Autodesk Inventor part; units mm, degrees
ref_plane "YZ Plane" through (0, 0, 0) normal (1, 0, 0) x (0, 1, 0)
ref_plane "XZ Plane" through (0, 0, 0) normal (0, 1, 0) x (-1, 0, 0)
ref_plane "XY Plane" through (0, 0, 0) normal (0, 0, 1) x (1, 0, 0)
sketch "TFT LCD Touch Screen" plane through (0, 0, 0) normal (0, 0, 1) x (1, 0, 0)
  line L0 (-55, 32.5) -> (55, 32.5)
  line L1 (55, 32.5) -> (55, -32.5)
  line L2 (55, -32.5) -> (-55, -32.5)
  line L3 (-55, -32.5) -> (-55, 32.5)
  circle A0 centre (-51, 28.5) radius 1.5
  circle A1 centre (-51, -28.5) radius 1.5
  circle A2 centre (51, -28.5) radius 1.5
  circle A3 centre (51, 28.5) radius 1.5
  line L4 (-40, 29) -> (40, 29)
  line L5 (40, 29) -> (40, -29)
  line L6 (40, -29) -> (-40, -29)
  line L7 (-40, -29) -> (-40, 29)
  point P0 (0.75, 3.075)
  point P1 (0, 32.5)
  point P2 (55, 0)
  point P3 (0, 29)
  point P4 (-40, 0)
  dimension "d9" = 110
  dimension "d10" = 65
  dimension "d11" = 3
  dimension "d12" = 57
  dimension "d13" = 102
  dimension "d14" = 4
  dimension "d15" = 4
  dimension "d16" = 80
  dimension "d17" = 58
sketch "Hinges Screw Holes" plane through (0, 0, 0) normal (0, 0, 1) x (1, 0, 0)
  arc A0 (172, 94.429) -> (172, 97.929) centre (172, 96.179) ccw
  arc A1 (172, 68.929) -> (172, 72.429) centre (172, 70.679) ccw
  arc A2 (172, -27.2) -> (172, -23.7) centre (172, -25.45) ccw
  arc A3 (172, -52.7) -> (172, -49.2) centre (172, -50.95) ccw
  arc A4 (167, 97.929) -> (167, 94.429) centre (167, 96.179) ccw
  arc A5 (167, 72.429) -> (167, 68.929) centre (167, 70.679) ccw
  arc A6 (167, -23.7) -> (167, -27.2) centre (167, -25.45) ccw
  arc A7 (167, -49.2) -> (167, -52.7) centre (167, -50.95) ccw
  line L0 (167, 97.929) -> (172, 97.929)
  line L1 (167, 94.429) -> (172, 94.429)
  line L2 (167, 72.429) -> (172, 72.429)
  line L3 (167, 68.929) -> (172, 68.929)
  line L4 (167, -23.7) -> (172, -23.7)
  line L5 (167, -27.2) -> (172, -27.2)
  line L6 (167, -49.2) -> (172, -49.2)
  line L7 (167, -52.7) -> (172, -52.7)
  point P0 (169.5, 0)
  point P1 (0, -7.5)
  dimension "d47" = 3.5
  dimension "d48" = 3.5
  dimension "d50" = 25.5
  dimension "d51" = 3.5
  dimension "d52" = 3.5
  dimension "d53" = 25.5
  dimension "d58" = 3.5
  dimension "d59" = 3.5
  dimension "d60" = 25.5
  dimension "d61" = 3.5
  dimension "d62" = 3.5
  dimension "d63" = 25.5
  dimension "d65" = 5
  dimension "d70" = 78.179
  dimension "d71" = 17.95
sketch "Door Shape" plane through (0, 0, 0) normal (0, 0, 1) x (1, 0, 0)
  line L0 (182, -55.7) -> (182, 113)
  line L1 (182, 113) -> (162, 133)
  line L2 (162, 133) -> (-162, 133)
  line L3 (-162, 133) -> (-182, 113)
  line L4 (-182, 113) -> (-182, -114)
  line L5 (-182, -114) -> (-162, -134)
  line L6 (-162, -134) -> (13.05, -134)
  line L7 (13.05, -134) -> (33.05, -114)
  line L8 (33.05, -114) -> (33.05, -55.7)
  line L9 (33.05, -55.7) -> (182, -55.7)
  line L10 (-161.8343, 132.6) -> (161.8343, 132.6)
  line L11 (161.8343, 132.6) -> (181.6, 112.8343)
  line L12 (181.6, 112.8343) -> (181.6, -55.3)
  line L13 (181.6, -55.3) -> (32.65, -55.3)
  line L14 (32.65, -55.3) -> (32.65, -113.8343)
  line L15 (32.65, -113.8343) -> (12.8843, -133.6)
  line L16 (12.8843, -133.6) -> (-161.8343, -133.6)
  line L17 (-161.8343, -133.6) -> (-181.6, -113.8343)
  line L18 (-181.6, -113.8343) -> (-181.6, 112.8343)
  line L19 (-181.6, 112.8343) -> (-161.8343, 132.6)
  line L20 (12.8843, -133.6) -> (181.6, -133.6)
  line L21 (181.6, -133.6) -> (181.6, -55.3)
  point P0 (-8.285, -11.54)
  dimension "d79" = 0.4
sketch "Sketch1" plane through (0, 0, 0) normal (0, 0, 1) x (1, 0, 0)
  line L0 (-182, 133.5) -> (182, 133.5)
  line L1 (182, 133.5) -> (182, -133.5)
  line L2 (182, -133.5) -> (-182, -133.5)
  line L3 (-182, -133.5) -> (-182, 133.5)
  line L4 (181.5, 133) -> (-181.5, 133)
  line L5 (-181.5, 133) -> (-181.5, -133)
  line L6 (-181.5, -133) -> (181.5, -133)
  line L7 (181.5, -133) -> (181.5, 133)
  point P0 (0, 0)
  point P1 (0, 133.5)
  point P2 (-181.5, 0)
  dimension "d0" = 364
  dimension "d1" = 267
  dimension "d4" = 0.5
extrude "Extrusion1" add sketch "Sketch1" along normal blind 2.8 contours L7 L6 L5 L4
chamfer "Chamfer1" distance 20 angle 45 4 edges at (-181.5, -133, 1.4) (-181.5, 133, 1.4) (181.5, -133, 1.4) (181.5, 133, 1.4)
fillet "Fillet1" radius 5 8 edges at (-161.5, -133, 1.4) (161.5, -133, 1.4) (181.5, -113, 1.4) (181.5, 113, 1.4) (161.5, 133, 1.4) (-161.5, 133, 1.4) (-181.5, 113, 1.4) (-181.5, -113, 1.4)
sketch "Sketch6" plane through (0, 0, 2.8) normal (0, 0, 1) x (1, 0, 0)
  line L0 (181.5, -110.9289) -> (181.5, 110.9289)
  arc A0 (172, 101.929) -> (172, 105.429) centre (172, 103.679) ccw
  arc A1 (172, 76.429) -> (172, 79.929) centre (172, 78.179) ccw
  arc A2 (172, -19.7) -> (172, -16.2) centre (172, -17.95) ccw
  arc A3 (172, -45.2) -> (172, -41.7) centre (172, -43.45) ccw
  arc A4 (167, 105.429) -> (167, 101.929) centre (167, 103.679) ccw
  arc A5 (167, 79.929) -> (167, 76.429) centre (167, 78.179) ccw
  arc A6 (167, -16.2) -> (167, -19.7) centre (167, -17.95) ccw
  arc A7 (167, -41.7) -> (167, -45.2) centre (167, -43.45) ccw
  line L1 (167, 105.429) -> (172, 105.429)
  line L2 (167, 101.929) -> (172, 101.929)
  line L3 (167, 79.929) -> (172, 79.929)
  line L4 (167, 76.429) -> (172, 76.429)
  line L5 (167, -16.2) -> (172, -16.2)
  line L6 (167, -19.7) -> (172, -19.7)
  line L7 (167, -41.7) -> (172, -41.7)
  line L8 (167, -45.2) -> (172, -45.2)
  point P0 (0, 0)
  dimension "d68" = 9.5
  dimension "d69" = 9.5
  dimension "d72" = 78.179
extrude "Extrusion5" cut sketch "Sketch6" against normal blind 10
sketch "Sketch7" plane through (0, 0, 2.8) normal (0, 0, 1) x (1, 0, 0)
  circle A0 centre (-161.5, 40) radius 1.75
  circle A1 centre (-161.5, -40) radius 1.75
  line L0 (-181.5, 110.9289) -> (-181.5, -110.9289)
  point P0 (0, 0)
  dimension "d73" = 3.5
  dimension "d74" = 80
  dimension "d75" = 40
  dimension "d76" = 20
extrude "Extrusion6" cut sketch "Sketch7" against normal blind 18.5
sketch "Sketch8" plane through (0, 0, 2.8) normal (0, 0, 1) x (1, 0, 0)
  line L0 (-181.5, 110.9289) -> (-181.5, -110.9289)
  line L1 (159.4289, 133) -> (-159.4289, 133)
  line L2 (182, -55.2) -> (182, 113.5)
  line L3 (182, 113.5) -> (162, 133.5)
  line L4 (162, 133.5) -> (-162, 133.5)
  line L5 (-162, 133.5) -> (-182, 113.5)
  line L6 (-182, 113.5) -> (-182, -113.5)
  line L7 (-182, -113.5) -> (-162, -133.5)
  line L8 (-162, -133.5) -> (13.05, -133.5)
  line L9 (13.05, -133.5) -> (33.05, -113.5)
  line L10 (33.05, -113.5) -> (33.05, -55.2)
  line L11 (33.05, -55.2) -> (182, -55.2)
  line L12 (-161.8343, 133.1) -> (161.8343, 133.1)
  line L13 (161.8343, 133.1) -> (181.6, 113.3343)
  line L14 (181.6, 113.3343) -> (181.6, -54.8)
  line L15 (181.6, -54.8) -> (32.65, -54.8)
  line L16 (32.65, -54.8) -> (32.65, -113.3343)
  line L17 (32.65, -113.3343) -> (12.8843, -133.1)
  line L18 (12.8843, -133.1) -> (-161.8343, -133.1)
  line L19 (-161.8343, -133.1) -> (-181.6, -113.3343)
  line L20 (-181.6, -113.3343) -> (-181.6, 113.3343)
  line L21 (-181.6, 113.3343) -> (-161.8343, 133.1)
  line L22 (12.8843, -133.1) -> (181.6, -133.1)
  line L23 (181.6, -133.1) -> (181.6, -54.8)
  point P0 (0, 0)
  point P1 (-182, 0)
  point P2 (-181.5, 0)
  point P3 (0, 133)
  point P4 (0, 133.5)
extrude "Extrusion7" cut sketch "Sketch8" against normal blind 18.5 contours L23 L22 L9 L10 L11 | L11 L10 L9 L22 L17 L16 L15 L23
fillet "Fillet3" radius 5 4 edges at (12.9843, -133, 1.4) (32.65, -113.3343, 1.4) (32.65, -54.8, 1.4) (181.5, -54.8, 1.4)
equation "\"d14\" = -0.5 * d12 + 0.5 * d10"
equation "\"d15\" = -0.5 * d13 + 0.5 * d9"
properties part number "Clear Front Door 2" material "Glass"
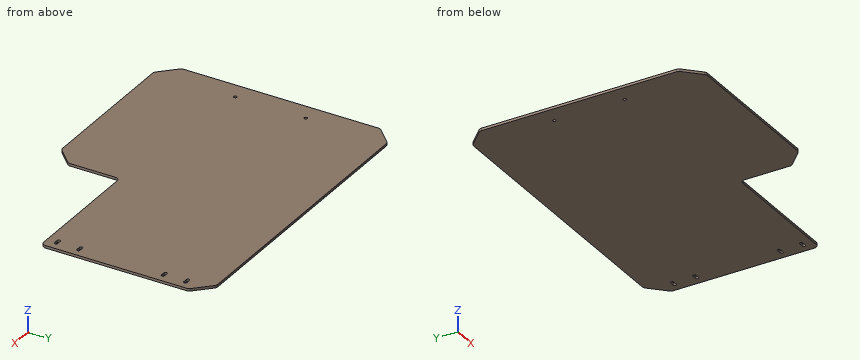
Geometry check sheet. Reference: the model listing, model coordinates, mm. Give positions to 0.01 mm unless a question says otherwise; leave off trailing zeros. Loops run counter-clockwise (first coordinate to the right, second up) from the corner with the lowest first, then second, coordinate; pieces in that order, holes last. Notation, with made-up numbers: (15.25, 71.25) -> (70.25, 71.25) arc R9 ccw to (70.25, 87.25) -> close; hole circle Ø11 at (-1, 8). An arc over 180 degrees is marked (long way). Answer in a Markdown table with one row per item. Add a question column.
1) Gauge pin test, flat ends, axial feed: P1, Ø0.8, axis at x = 170, z = 1, coming from the +Y side; P2, Ø0.8, axis at x = 168.5, z = 1.5, coming from the -Y side. Record the tip position at first contact, or that the pin passes through.
2) Material ranges on probe 1 along Y at (x, z) = (-161.5, 1.35); probe 2 along X at (y, z) = (-84.5, 1.3); probe 3 along Y at (x, z) = (98.5, 2.75), recorded low to high. Write a range as from..to.
3) Cross-section at A-A on x = 103.5. Record the boundary of the cut face in (y, z), and give its area (3 significant figures).
4) Cross-section at B-B on z = 2.1. State how many separate pieces and enclosed holes the cut face has, and give its area (3 significant figures).
Outcome:
| question | item | result |
|---|---|---|
| 1 | P1 | stops at y = 124.9 |
| 1 | P2 | stops at y = -54.8 |
| 2 | probe 1 | y = -132.55..-41.75, -38.25..38.25, 41.75..132.55 |
| 2 | probe 2 | x = -181.5..32.65 |
| 2 | probe 3 | y = -54.8..133 |
| 3 | outline | (-54.8, 0) -> (133, 0) -> (133, 2.8) -> (-54.8, 2.8) -> close |
| 3 | area | 526 mm^2 |
| 4 | separate pieces | 1 |
| 4 | enclosed holes | 6 |
| 4 | area | 84,000 mm^2 |
